The listing builds one solid part. Answer for the finished solid, in the listing's coordinates (mm). A direction names the side the tool comes from. Give positions to 0.01 mm unless a question says otherwise; leave off trailing zeros. Answer in a Markdown table with one row per item.
from build123d import *
from OCP.BRepAlgoAPI import BRepAlgoAPI_Cut
from OCP.TopTools import TopTools_ListOfShape

# Parameters (mm, degrees)
SKETCH1_R           = 15
SKETCH1_R_2         = 4.5
BOSS_EXTRUDE1_DEPTH = 1
BOSS_EXTRUDE2_START = -3.5
SKETCH1_2_R         = 4.5
BOSS_EXTRUDE2_DEPTH = 4.5
SKETCH2_R           = 1.5
CUT_EXTRUDE1_DEPTH  = 4.5
CUT_EXTRUDE2_START  = -4.5
SKETCH3_R           = 2.75
CUT_EXTRUDE2_DEPTH  = 3.5
CUT_EXTRUDE3_START  = -4.5
CUT_EXTRUDE3_DEPTH  = 3.5
CIRPATTERN1_COUNT   = 25
CUT_EXTRUDE4_START  = 9.886861
SKETCH6_R           = 1.5
CUT_EXTRUDE4_DEPTH  = 3.863123


with BuildPart() as part:
    # Sketch1 → Boss-Extrude1 (new body)
    with BuildSketch(Plane.XY):
        Circle(SKETCH1_R)
        Circle(SKETCH1_R_2, mode=Mode.SUBTRACT)
    extrude(amount=BOSS_EXTRUDE1_DEPTH)

    # Sketch1<2> → Boss-Extrude2 (add)
    with BuildSketch(Plane.XY.offset(BOSS_EXTRUDE2_START)):
        Circle(SKETCH1_2_R)
    extrude(amount=BOSS_EXTRUDE2_DEPTH)

    # Sketch2 → Cut-Extrude1 (cut)
    with BuildSketch(Plane(origin=(0, 0, 0), x_dir=(-1, 0, 0), z_dir=(0, 0, -1))):
        with Locations(Location((0, 0, 0), (0, 0, 180))):
            Circle(SKETCH2_R)
    extrude(amount=CUT_EXTRUDE1_DEPTH, mode=Mode.SUBTRACT)

    # Sketch3 → Cut-Extrude2 (cut)
    with BuildSketch(Plane(origin=(0, 0, -3.5), x_dir=(-1, 0, 0), z_dir=(0, 0, -1)).offset(CUT_EXTRUDE2_START)):
        with Locations(Location((0, 0, 0), (0, 0, 180))):
            Circle(SKETCH3_R)
    extrude(amount=CUT_EXTRUDE2_DEPTH, mode=Mode.SUBTRACT)

    # Sketch4 → Cut-Extrude3 (cut)
    with BuildSketch(Plane(origin=(0, 0, -3.5), x_dir=(-1, 0, 0), z_dir=(0, 0, -1)).offset(CUT_EXTRUDE3_START)):
        with BuildLine():
            Line((-2.665974712, 0.674595311), (-2.976344104, 0.375999701))
            Line((-2.976344104, 0.375999701), (-2.728315429, 0.344666392))
            ThreePointArc((-2.728315429, 0.344666392), (-2.70218519, 0.510583192), (-2.665974712, 0.674595311))
        make_face()
        with BuildLine():
            Line((-2.976344104, 0.375999701), (-2.75, 0))
            ThreePointArc((-2.75, 0), (-2.744573503, 0.172673929), (-2.728315429, 0.344666392))
            Line((-2.728315429, 0.344666392), (-2.976344104, 0.375999701))
        make_face()
    cut_extrude3 = extrude(amount=CUT_EXTRUDE3_DEPTH, mode=Mode.SUBTRACT)

    # CirPattern1: Cut-Extrude3 ×25 about axis
    cirpattern1_axis = Axis((0, 0, 0), (0, 0, 1))
    for i in range(1, CIRPATTERN1_COUNT):
        add(cut_extrude3.rotate(cirpattern1_axis, i * 360 / CIRPATTERN1_COUNT), mode=Mode.SUBTRACT)

    # Sketch5 → Revolve1 (revolve)
    with BuildSketch(Plane(origin=(0, 0, 0), x_dir=(1, 0, 0), z_dir=(0, 1, 0))):
        Polygon((-15, 0), (-12.5, 1.5), (-12.5, 3), (-15, 4.5), (-15, 5.5), (-10, 5.5), (-10, 0), align=None)
    revolve(axis=Axis((0, 0, -2.5), (0, 0, 1)))


with BuildPart() as cut_extrude4_tool:
    # Sketch6 → Cut-Extrude4 (new body)
    with BuildSketch(Plane(origin=(0, 0, 0), x_dir=(1, 0, 0), z_dir=(0, 1, 0)).offset(CUT_EXTRUDE4_START)):
        with Locations((0, 2.25)):
            Circle(SKETCH6_R)
    extrude(amount=CUT_EXTRUDE4_DEPTH)


with BuildPart() as part_1:
    add(part.part)

    # Cut-Extrude4: cut by cut_extrude4_tool, with a tolerance
    cut_extrude4_stock = TopTools_ListOfShape()
    cut_extrude4_stock.Append(part_1.part.wrapped)
    cut_extrude4_tools = TopTools_ListOfShape()
    cut_extrude4_tools.Append(cut_extrude4_tool.part.wrapped)
    cut_extrude4_cut = BRepAlgoAPI_Cut()
    cut_extrude4_cut.SetArguments(cut_extrude4_stock)
    cut_extrude4_cut.SetTools(cut_extrude4_tools)
    cut_extrude4_cut.SetFuzzyValue(0.00001)
    cut_extrude4_cut.Build()
    add(Compound.cast(cut_extrude4_cut.Shape()).solids(), mode=Mode.REPLACE)


solid = part_1.part
Item 1: Which of the six approach directions +Z, -Z, +X, -X, +Y, -Y give full straight-line access (tool end or side, diameter ignored) to faces 1 (the face through (-1.5, 11.4, -2.3)), 2 (the face through (-1.4, -1.4, -2.5)), 3 (the face through (-0.53, -12.49, -2.26)), 4 (the face through (4.3, -2.1, 0))?
Answer block:
| item | result |
|---|---|
| face 1 | +Y |
| face 2 | +Z |
| face 3 | none |
| face 4 | -Z |
Item 2: Each of these flat-tipped pins is pushed along its axis until it touches: P1, Ø2, axis at y = 6, z = -2.5, coming from the +X side; P2, Ø3.5, axis at x = 0, z = -2.25, coming from the +Y side; P3, Ø1.5, axis at x = -4, z = 0, coming from the -Y side. Where does it stop, or does it pass through?
Answer block:
| item | result |
|---|---|
| P1 | x = 11.97 |
| P2 | y = 14.17 |
| P3 | y = -14.64 |
Item 3: Consider line 1 (Y direction, x = 0, z = -2.65); line 2 (Y direction, x = -1, z = -0.75); line 3 (X direction, y = 6, z = -0.75). Determine where each line is inside the solid, lowest interval first.
Answer block:
| item | result |
|---|---|
| line 1 | -12.5 to -10, -4.5 to -1.5, 1.5 to 4.5 |
| line 2 | -13.71 to -9.95, -4.39 to -2.74, 2.74 to 4.39, 9.95 to 13.71 |
| line 3 | -12.37 to -8, 8 to 12.37 |
Item 4: Determine the mould class of faces 5 (the face through (-14.985, 0.66, 0.493)), 6 (the face through (-0.59, 4.46, -1.77)), 7 (the face through (3, 0, 1)) for opening direction X: pulls with the +X half, pulls with the -X half, needs draft (parallel to the pull), parting line crosses it, or undercut.
Answer block:
| item | result |
|---|---|
| face 5 | parting line crosses it |
| face 6 | undercut |
| face 7 | needs draft |
